```python
from build123d import *

# Parameters (mm, degrees)
SKETCH_11_W         = 15
SKETCH_11_H         = 15
SKETCH_11_W_2       = 13
SKETCH_11_H_2       = 13
F_15X15X1_1_DEPTH   = 615
SKETCH_12_R         = 1.45
CUT_EXTRUDE_1_DEPTH = 616.228616044
SKETCH_13_R         = 1.45
CUT_EXTRUDE_2_DEPTH = 616.228616044
SKETCH_14_R         = 1.45
CUT_EXTRUDE_3_DEPTH = 616.228616044


with BuildPart() as part:
    # 草图11 → 铝管 15X15X1(1) (new body)
    with BuildSketch(Plane.ZY):
        Rectangle(SKETCH_11_W, SKETCH_11_H)
        Rectangle(SKETCH_11_W_2, SKETCH_11_H_2, mode=Mode.SUBTRACT)
    extrude(amount=F_15X15X1_1_DEPTH)

    # 草图12 → 切除-拉伸1 (cut, through all)
    with BuildSketch(Plane(origin=(0, 7.5, 0), x_dir=(1, 0, 0), z_dir=(0, 1, 0))):
        with Locations(Location((-610, 0, 0), (0, 0, 270))):
            Circle(SKETCH_12_R)
        with Locations(Location((-590, 0, 0), (0, 0, 270))):
            Circle(SKETCH_12_R)
        with Locations(Location((-25, 0, 0), (0, 0, 90))):
            Circle(SKETCH_12_R)
        with Locations(Location((-5, 0, 0), (0, 0, 90))):
            Circle(SKETCH_12_R)
    extrude(amount=-CUT_EXTRUDE_1_DEPTH, mode=Mode.SUBTRACT)

    # 草图13 → 切除-拉伸2 (cut, through all)
    with BuildSketch(Plane.XZ.offset(7.5)):
        with Locations(Location((-102.5, 0, 0), (0, 0, 270))):
            Circle(SKETCH_13_R)
        with Locations(Location((-72.5, 0, 0), (0, 0, 270))):
            Circle(SKETCH_13_R)
        with Locations(Location((-42.5, 0, 0), (0, 0, 270))):
            Circle(SKETCH_13_R)
        with Locations(Location((-542.5, 0, 0), (0, 0, 270))):
            Circle(SKETCH_13_R)
        with Locations(Location((-512.5, 0, 0), (0, 0, 270))):
            Circle(SKETCH_13_R)
        with Locations(Location((-572.5, 0, 0), (0, 0, 270))):
            Circle(SKETCH_13_R)
    extrude(amount=-CUT_EXTRUDE_2_DEPTH, mode=Mode.SUBTRACT)

    # 草图14 → 切除-拉伸3 (cut, through all)
    with BuildSketch(Plane.XZ.offset(7.5)):
        with Locations(Location((-492.5, 0, 0), (0, 0, 270))):
            Circle(SKETCH_14_R)
        with Locations(Location((-482.5, 0, 0), (0, 0, 270))):
            Circle(SKETCH_14_R)
        with Locations(Location((-472.5, 0, 0), (0, 0, 270))):
            Circle(SKETCH_14_R)
        with Locations(Location((-462.5, 0, 0), (0, 0, 270))):
            Circle(SKETCH_14_R)
        with Locations(Location((-452.5, 0, 0), (0, 0, 270))):
            Circle(SKETCH_14_R)
        with Locations(Location((-442.5, 0, 0), (0, 0, 270))):
            Circle(SKETCH_14_R)
        with Locations(Location((-432.5, 0, 0), (0, 0, 270))):
            Circle(SKETCH_14_R)
        with Locations(Location((-422.5, 0, 0), (0, 0, 270))):
            Circle(SKETCH_14_R)
        with Locations(Location((-412.5, 0, 0), (0, 0, 270))):
            Circle(SKETCH_14_R)
        with Locations(Location((-402.5, 0, 0), (0, 0, 270))):
            Circle(SKETCH_14_R)
        with Locations(Location((-392.5, 0, 0), (0, 0, 270))):
            Circle(SKETCH_14_R)
        with Locations(Location((-382.5, 0, 0), (0, 0, 270))):
            Circle(SKETCH_14_R)
        with Locations(Location((-372.5, 0, 0), (0, 0, 270))):
            Circle(SKETCH_14_R)
        with Locations(Location((-362.5, 0, 0), (0, 0, 270))):
            Circle(SKETCH_14_R)
        with Locations(Location((-352.5, 0, 0), (0, 0, 270))):
            Circle(SKETCH_14_R)
        with Locations(Location((-342.5, 0, 0), (0, 0, 270))):
            Circle(SKETCH_14_R)
        with Locations(Location((-332.5, 0, 0), (0, 0, 270))):
            Circle(SKETCH_14_R)
        with Locations(Location((-322.5, 0, 0), (0, 0, 270))):
            Circle(SKETCH_14_R)
        with Locations(Location((-312.5, 0, 0), (0, 0, 270))):
            Circle(SKETCH_14_R)
        with Locations(Location((-302.5, 0, 0), (0, 0, 270))):
            Circle(SKETCH_14_R)
        with Locations(Location((-292.5, 0, 0), (0, 0, 270))):
            Circle(SKETCH_14_R)
        with Locations(Location((-282.5, 0, 0), (0, 0, 270))):
            Circle(SKETCH_14_R)
        with Locations(Location((-272.5, 0, 0), (0, 0, 270))):
            Circle(SKETCH_14_R)
        with Locations(Location((-262.5, 0, 0), (0, 0, 270))):
            Circle(SKETCH_14_R)
        with Locations(Location((-252.5, 0, 0), (0, 0, 270))):
            Circle(SKETCH_14_R)
        with Locations(Location((-242.5, 0, 0), (0, 0, 270))):
            Circle(SKETCH_14_R)
        with Locations(Location((-232.5, 0, 0), (0, 0, 270))):
            Circle(SKETCH_14_R)
        with Locations(Location((-222.5, 0, 0), (0, 0, 270))):
            Circle(SKETCH_14_R)
        with Locations(Location((-212.5, 0, 0), (0, 0, 270))):
            Circle(SKETCH_14_R)
        with Locations(Location((-202.5, 0, 0), (0, 0, 270))):
            Circle(SKETCH_14_R)
        with Locations(Location((-192.5, 0, 0), (0, 0, 270))):
            Circle(SKETCH_14_R)
        with Locations(Location((-182.5, 0, 0), (0, 0, 270))):
            Circle(SKETCH_14_R)
        with Locations(Location((-172.5, 0, 0), (0, 0, 270))):
            Circle(SKETCH_14_R)
        with Locations(Location((-162.5, 0, 0), (0, 0, 270))):
            Circle(SKETCH_14_R)
        with Locations(Location((-152.5, 0, 0), (0, 0, 270))):
            Circle(SKETCH_14_R)
        with Locations(Location((-142.5, 0, 0), (0, 0, 270))):
            Circle(SKETCH_14_R)
        with Locations(Location((-132.5, 0, 0), (0, 0, 270))):
            Circle(SKETCH_14_R)
        with Locations(Location((-122.5, 0, 0), (0, 0, 270))):
            Circle(SKETCH_14_R)
        with Locations(Location((-112.5, 0, 0), (0, 0, 270))):
            Circle(SKETCH_14_R)
    extrude(amount=-CUT_EXTRUDE_3_DEPTH, mode=Mode.SUBTRACT)


solid = part.part
```
Could you check a few things on this model? Use its own coordinates, in mm. A direction names the side the tool comes from. Coordinates: 2 decimals unless noted, no trailing zeros. Write each loop counter-clockwise with the first axis right and the second up, starting at its lowest first coordinate (ties: lowest second). Pieces come first, ordered by that corner, then holes. Notation, with made-up numbers: (43.25, 87.5) -> (58.25, 87.5) arc R29 cw to (58.25, 107.5) -> close; hole circle Ø9 at (80, 13). An arc over 180 degrees is marked (long way). Write item = value, one per line. Start each with the question number.
(1) Will these pins go through, and if not, where does the flat tip stop? pin 1 (3.5 mm diameter, centred on x = -332.5, z = 0, fed in from +Y); pin 2 (2.5 mm diameter, centred on x = -312.5, z = 0, fed in from +Y).
(2) I need wall thicknesses on line 1 (Y direction, x = -45.5, z = 6); line 2 (Z direction, x = -172.5, y = -7.15). Which ranges of each line are inside material? Lowest first, please. Write a range as [from, to].
(3) I want a section at B-B (y = -1). Please give me the cut outline in (x, z), plus the area to 3 significant figures.
(4) We'd pull the mould along Y, two halves only. Please class faces 1 (the face through (-303, -7.5, -2)), 2 (the face through (-303, 6.5, -2)), 3 (the face through (-303, 0, 7.5)), 4 (the face through (-303, 0, 6.5)): released by +Y, released by -Y, zero draft, split by the parting line, or undercut.
(5) I want a section at A-A (x = -506). Please give me the cut outline in (y, z), plus the area to 3 significant figures.
(6) Which directions (+Z, -Z, +X, -X, +Y, -Y) give clear straight access to the entire face, cutting with the end or side of a thin tool? Please do faces 5 (the face through (-303, 0, -6.5)), 6 (the face through (-615, 0, -7)).
Result set:
q1.pin_1 = 7.5
q1.pin_2 = through
q2.line_1 = [-7.5, -6.5], [6.5, 7.5]
q2.line_2 = [-7.5, -1.45], [1.45, 7.5]
q3.outline = (-615, -7.5) -> (0, -7.5) -> (0, -6.5) -> (-615, -6.5) -> close; (-615, 6.5) -> (0, 6.5) -> (0, 7.5) -> (-615, 7.5) -> close
q3.area = 1,230 mm2
q4.face_1 = released by -Y
q4.face_2 = undercut
q4.face_3 = zero draft
q4.face_4 = undercut
q5.outline = (-7.5, -7.5) -> (7.5, -7.5) -> (7.5, 7.5) -> (-7.5, 7.5) -> close; hole (-6.5, -6.5) -> (6.5, -6.5) -> (6.5, 6.5) -> (-6.5, 6.5) -> close
q5.area = 56.0 mm2
q6.face_5 = +X, -X
q6.face_6 = +Z, -Z, -X, +Y, -Y
